Part model, mm, in its own coordinate system. A direction names the side the tool comes from. Round coordinates to 2 decimals unless told otherwise and drop trailing zeros. Order: outer loops, then holes, each group sorted by start corner. A loop starts at its lowest first (then second) coordinate and runs counter-clockwise, first axis right, second up. Notation, with made-up numbers: (48, 80) -> (100, 80) arc R34 cw to (100, 115) -> close; hole circle Ø2 at (58, 17). An arc over 180 degrees is marked (long way). Answer as a JSON object with one key per item and string values. Group by question number.
```python
from build123d import *

# Parameters (mm, degrees)
SKETCH_W          = 70
SKETCH_H          = 100
PAD_DEPTH         = 3
SKETCH001_W       = 64
SKETCH001_H       = 94
PAD001_DEPTH      = 3
PAD001_DEPTH_BACK = 10
SKETCH002_W       = 54
SKETCH002_H       = 84
POCKET_DEPTH      = 11
SKETCH003_R       = 3.175
POCKET001_DEPTH   = 2.001
FILLET_R          = 5
FILLET001_R       = 5
FILLET002_R       = 5
FILLET003_R       = 5
FILLET004_R       = 1


with BuildPart() as part:
    # Sketch → Pad (new body)
    with BuildSketch(Plane.XY):
        with Locations((35, 50)):
            Rectangle(SKETCH_W, SKETCH_H)
    extrude(amount=PAD_DEPTH)

    # Sketch001 (on Face6 of Pad) → Pad001 (join, two sides)
    with BuildSketch(Plane.XY.offset(3)) as pad001_sk:
        with Locations((35, 50)):
            Rectangle(SKETCH001_W, SKETCH001_H)
    extrude(amount=PAD001_DEPTH)
    extrude(pad001_sk.sketch, amount=-PAD001_DEPTH_BACK)

    # Sketch002 (on Face16 of Pad001) → Pocket (cut)
    with BuildSketch(Plane.XY.offset(6)):
        with Locations((35, 50)):
            Rectangle(SKETCH002_W, SKETCH002_H)
    extrude(amount=-POCKET_DEPTH, mode=Mode.SUBTRACT)

    # Sketch003 (on Face21 of Pocket) → Pocket001 (cut, through all)
    with BuildSketch(Plane.XY.offset(-5)):
        with Locations((50, 30)):
            Circle(SKETCH003_R)
        with Locations((50, 70)):
            Circle(SKETCH003_R)
        with BuildLine():
            ThreePointArc((21.775097, 28.4), (28.6, 30), (21.775097, 31.6))
            Line((16.7, 31.6), (21.775097, 31.6))
            Line((16.7, 28.4), (16.7, 31.6))
            Line((21.775097, 28.4), (16.7, 28.4))
        make_face()
        with BuildLine():
            ThreePointArc((21.775097, 68.4), (28.6, 70), (21.775097, 71.6))
            Line((16.7, 71.6), (21.775097, 71.6))
            Line((16.7, 68.4), (16.7, 71.6))
            Line((21.775097, 68.4), (16.7, 68.4))
        make_face()
    extrude(amount=-POCKET001_DEPTH, mode=Mode.SUBTRACT)

    # Fillet
    fillet_edges = [part.edges().sort_by_distance(p)[0] for p in [
        (3, 3, 4.5),
    ]]
    fillet(fillet_edges, radius=FILLET_R)

    # Fillet001
    fillet001_edges = [part.edges().sort_by_distance(p)[0] for p in [
        (67, 3, 4.5),
    ]]
    fillet(fillet001_edges, radius=FILLET001_R)

    # Fillet002
    fillet002_edges = [part.edges().sort_by_distance(p)[0] for p in [
        (67, 97, 4.5),
    ]]
    fillet(fillet002_edges, radius=FILLET002_R)

    # Fillet003
    fillet003_edges = [part.edges().sort_by_distance(p)[0] for p in [
        (3, 97, 4.5),
    ]]
    fillet(fillet003_edges, radius=FILLET003_R)

    # Fillet004
    fillet004_edges = [part.edges().sort_by_distance(p)[0] for p in [
        (35, 97, 6),
    ]]
    fillet(fillet004_edges, radius=FILLET004_R)


solid = part.part
```
Q1. Wall check: line 1 (Y direction, x = 50, z = -6.1) (3 decimals); line 2 (Y direction, x = 25, z = -5.5); line 3 (X direction, y = 29, z = -3). Give the ranges that are in metal, low to high. Write a range as [from, to].
Q2. Band-saw the part on C-C (z = -4). List the corners of the cut face in (x, y), plus the area to 3 significant figures.
Q3. Band-saw the part on A-A (x = 25). List the corners of the cut face in (y, z), plus the area to 3 significant figures.
Q4. Drop flat-ended pins along their axis: pin 1 Ø4.5 at (x, y) = (25, 30) entering from -Z; pin 2 Ø3 at (x, y) = (55, 44.5) entering from +Z; pin 3 Ø0.6 at (y, z) = (70.5, -6.5) entering from +X; pin 4 Ø4 at (x, z) = (39, -5.5) entering from -Y. Give the stop position or say it passes through.
Q5. Which spindle directions (+Z, -Z, +X, -X, +Y, -Y) get a long thin tool onto all of the face, cutting with end or side? Do faces 5 (the flat face through (35, 97, -3)), 6 (the flat face through (16.7, 30, -6)), 7 (the flat face through (67, 49, 4)), 8 (the flat face through (35, 8, 1)). Say none if no direction does.
Q6. Two-plate mould, pull along X, no slides. Class faces 1 (the cylindrical face through (28.6, 69.9, -6)), 2 (the flat face through (7, 54, 6)), 3 (the flat face through (62, 49, 1)), 4 (the cylindrical face through (66, 95, 4)): +X half, -X half, draft (parallel to the pull), parting line (faces both ways), or undercut.
Q7. Band-saw the part on B-B (y = 70). List the corners of the cut face in (x, z) (3 decimals), plus the area to 3 significant figures.
Q8. Band-saw the part on D-D (x = 33). List the corners of the cut face in (y, z).
Completed:
{
 "1": {"line 1": "[3, 26.825], [33.175, 66.825], [73.175, 97]", "line 2": "[3, 26.4], [33.6, 66.4], [73.6, 97]", "line 3": "[3, 8], [62, 67]"},
 "2": {"outline": "(3, 3) -> (67, 3) -> (67, 97) -> (3, 97) -> close; hole (8, 8) -> (62, 8) -> (62, 92) -> (8, 92) -> close", "area": "1,480 mm2"},
 "3": {"outline": "(0, 0) -> (3, 0) -> (3, -7) -> (26.4, -7) -> (26.4, -5) -> (8, -5) -> (8, 6) -> (4, 6) arc R1 ccw to (3, 5) -> (3, 3) -> (0, 3) -> close; (33.6, -7) -> (66.4, -7) -> (66.4, -5) -> (33.6, -5) -> close; (73.6, -7) -> (97, -7) -> (97, 0) -> (100, 0) -> (100, 3) -> (97, 3) -> (97, 5) arc R1 ccw to (96, 6) -> (92, 6) -> (92, -5) -> (73.6, -5) -> close", "area": "287 mm2"},
 "4": {"pin 1": "through", "pin 2": "z = -5", "pin 3": "x = 67", "pin 4": "y = 3"},
 "5": {"face 5": "-Z, +X, -X, +Y", "face 6": "+Z, -Z", "face 7": "+Z, +X, +Y, -Y", "face 8": "+Z"},
 "6": {"face 1": "undercut", "face 2": "draft", "face 3": "undercut", "face 4": "+X half"},
 "7": {"outline": "(0, 0) -> (3, 0) -> (3, -7) -> (16.7, -7) -> (16.7, -5) -> (8, -5) -> (8, 6) -> (4, 6) arc R1 ccw to (3, 5) -> (3, 3) -> (0, 3) -> close; (28.6, -7) -> (46.825, -7) -> (46.825, -5) -> (28.6, -5) -> close; (53.175, -7) -> (67, -7) -> (67, 0) -> (70, 0) -> (70, 3) -> (67, 3) -> (67, 5) arc R1 ccw to (66, 6) -> (62, 6) -> (62, -5) -> (53.175, -5) -> close", "area": "219 mm2"},
 "8": {"outline": "(0, 0) -> (3, 0) -> (3, -7) -> (97, -7) -> (97, 0) -> (100, 0) -> (100, 3) -> (97, 3) -> (97, 5) arc R1 ccw to (96, 6) -> (92, 6) -> (92, -5) -> (8, -5) -> (8, 6) -> (4, 6) arc R1 ccw to (3, 5) -> (3, 3) -> (0, 3) -> close"}
}
